from build123d import *

# Parameters (mm, degrees)
ESQUISSE1_R             = 45
BASE_EXTRUSION_DEPTH    = 20
ESQUISSE2_R             = 30
ENL_V_MAT_EXTRU_1_DEPTH = 20
ESQUISSE3_W             = 30
ESQUISSE3_H             = 2
ENL_V_MAT_EXTRU_2_DEPTH = 20
ESQUISSE4_R             = 3
ENL_V_MAT_EXTRU_3_DEPTH = 103.591422643
ESQUISSE5_R             = 7
ENL_V_MAT_EXTRU_4_DEPTH = 40
CONG_1_R                = 2
ESQUISSE6_R             = 3
ENL_V_MAT_EXTRU_5_DEPTH = 20


with BuildPart() as part:
    # Esquisse1 → Base-Extrusion (new body)
    with BuildSketch(Plane.XY):
        Circle(ESQUISSE1_R)
    extrude(amount=BASE_EXTRUSION_DEPTH)

    # Esquisse2 → Enlèv. mat.-Extru.1 (cut)
    with BuildSketch(Plane.XY.offset(20)):
        Circle(ESQUISSE2_R)
    extrude(amount=-ENL_V_MAT_EXTRU_1_DEPTH, mode=Mode.SUBTRACT)

    # Esquisse3 → Enlèv. mat.-Extru.2 (cut)
    with BuildSketch(Plane.XY.offset(20)):
        with Locations((-35, 0)):
            Rectangle(ESQUISSE3_W, ESQUISSE3_H)
    extrude(amount=-ENL_V_MAT_EXTRU_2_DEPTH, mode=Mode.SUBTRACT)

    # Esquisse4 → Enlèv. mat.-Extru.3 (cut, through all)
    with BuildSketch(Plane(origin=(0, 45, 0), x_dir=(-1, 0, 0), z_dir=(0, 1, 0))):
        with Locations(Location((37.5, 10, 0), (0, 0, 90))):
            Circle(ESQUISSE4_R)
    extrude(amount=-ENL_V_MAT_EXTRU_3_DEPTH, mode=Mode.SUBTRACT)

    # Esquisse5 → Enlèv. mat.-Extru.4 (cut)
    with BuildSketch(Plane(origin=(0, 45, 0), x_dir=(-1, 0, 0), z_dir=(0, 1, 0))):
        with Locations(Location((37.5, 10, 0), (0, 0, 90))):
            Circle(ESQUISSE5_R)
    extrude(amount=-ENL_V_MAT_EXTRU_4_DEPTH, mode=Mode.SUBTRACT)

    # Congé1
    cong_1_edges = [part.edges().sort_by_distance(p)[0] for p in [
        (0.500030871, 44.997221793, 20),
        (0.500030871, -44.997221793, 20),
    ]]
    fillet(cong_1_edges, radius=CONG_1_R)

    # Esquisse6 → Enlèv. mat.-Extru.5 (cut)
    with BuildSketch(Plane.XY.offset(20)):
        with Locations((37.5, 0)):
            Circle(ESQUISSE6_R)
    extrude(amount=-ENL_V_MAT_EXTRU_5_DEPTH, mode=Mode.SUBTRACT)


solid = part.part
Verification items for the finished model (mm, model axes). A direction names the side the tool comes from. Coordinates: 2 decimals unless noted, no trailing zeros. Write each loop counter-clockwise with the first axis right and the second up, starting at its lowest first coordinate (ties: lowest second). Pieces come first, ordered by that corner, then holes. Notation, with made-up numbers: (9, 41) -> (21, 41) arc R15 cw to (21, 45) -> close; hole circle Ø3 at (-27.5, -4). An arc over 180 degrees is marked (long way). One line per item, written item: value. Start each with the question number.
Q1. Mould release check, pull along Y, two halves, no side actions. Record for faces 4 (the cylindrical face through (-34.97, 3.03, 11.61)), 5 (the flat face through (-41, 5, 10)), 6 (the cylindrical face through (34.5, 0.1, 10.1)): pulls with the +Y half, pulls with the -Y half, needs draft (parallel to the pull), parting line crosses it, or undercut.
Q2. Go/stop test with flat-tipped pins: P1, Ø8, axis at x = -31.5, z = 15.5, coming from the +Y side; P2, Ø5, axis at y = -30.5, z = 16.5, coming from the -X side; P3, Ø12, axis at x = -12, z = 11, coming from the -Y side; P4, Ø3.5, axis at x = -37.5, z = 10, coming from the +Y side. Record where each tip stops, or that it passes through.
Q3. Cross-section at A-A on x = 0. Enter the section's corners in (y, z).
Q4. Access from +Z, -Z, +X, -X, +Y, -Y to the whole of each face (thin tool, end or side, straight path). Record for faces 1 (the cylindrical face through (-30.56, 16.12, 9.09)), 2 (the cylindrical face through (-34.526, -11.652, 9.609)), 3 (the flat face through (-34, -1, 10)).
Q5. Cross-section at B-B on z = 10. Enter the section's corners in (x, y), and give its area (3 significant figures).
Q6. Thickness scan on L1, parallel to X at y = -12.5, z = 10; L2, parallel to Z at x = -37.5, y = 12.5; L3, parallel to X at y = 1.85, z = 10. Record the ranges inside material, lowest first. Write a range as from..to.
Q7. Cross-section at C-C on y = -18. State how many separate pieces and enclosed holes the cut face has, and give its area (3 significant figures).
Checked values:
1. face 4: needs draft
1. face 5: pulls with the +Y half
1. face 6: undercut
2. P1: stops at y = 35.62
2. P2: stops at x = -35.23
2. P3: stops at y = -44.6
2. P4: passes through
3. outline: (-45, 0) -> (-30, 0) -> (-30, 20) -> (-43, 20) arc R2 ccw to (-45, 18) -> close; (30, 0) -> (45, 0) -> (45, 18) arc R2 ccw to (43, 20) -> (30, 20) -> close
4. face 1: +Y
4. face 2: +Y, -Y
4. face 3: +Z, -Z, -X
5. outline: (-44.99, -1) arc R45 ccw to (-40.5, -19.62) -> (-40.5, -1) -> close; (-44.99, 1) -> (-40.5, 1) -> (-40.5, 5) -> (-44.5, 5) -> (-44.5, 6.69) arc R45 ccw to start; (-34.5, -28.89) arc R45 ccw (long way) to (-30.5, 33.09) -> (-30.5, 5) -> (-34.5, 5) -> (-34.5, 1) -> (-29.98, 1) arc R30 cw (long way) to (-29.98, -1) -> (-34.5, -1) -> close; hole circle Ø6 at (37.5, 0)
5. area: 3,050 mm²
6. L1: x = -43.23..-40.5, -34.5..-27.27, 27.27..43.23
6. L2: z = 0..3, 17..20
6. L3: x = -44.96..-40.5, -34.5..-29.94, 29.94..35.14, 39.86..44.96
7. separate pieces: 2
7. enclosed holes: 1
7. area: 660 mm²
